For this review, take the finished solid that the model builds, in its own axes (mm). A direction names the side the tool comes from. Give positions to 0.01 mm unless a question says otherwise; leave off trailing zeros. Write each loop counter-clockwise with the first axis right and the second up, starting at its lowest first coordinate (ties: lowest second). Pieces come first, ordered by that corner, then holes. Notation, with made-up numbers: M 34,62.25 L 86,62.25 A13 ccw 86,87.25 Z; hole C 33.5,43 d4. An arc over 180 degrees is marked long. One line per item, written item: value. Start each with the question number.
Item 1: Clearance check with flat-ended pins moving along their axes: pin 1 Ø10 at (x, z) = (59, 13.5) entering from -Y; pin 2 Ø21 at (x, y) = (31, 34) entering from -Z. State where each tip first meets the part, or that it passes through.
Item 2: Consider section A-A, the plane z = -2. Write out the cut boundary in (x, y).
Item 3: Consider section B-B, the plane x = 44. Write out the cut boundary in (y, z).
Item 4: Mouldability with a two-part tool opening along X and no side actions: class faces 6 (the face through (7, 6, -0.5)), 7 (the face through (36, 38, 25)) as released by +X, released by -X, zero draft, split by the parting line, or undercut.
Item 5: Consider section D-D, the plane y = 11. Write out the cut boundary in (x, z), and give its area (3 significant figures).
Item 6: To check wall thickness, follow probe 1 along Y at (x, z) = (66, -0.25); probe 2 along Z at (x, y) = (60.5, 46.5); probe 3 along X at (y, z) = (58.5, 6.5). State the ranges of each line that lie inside material, in increasing order.
Item 7: Tool access review of faces 1 (the face through (37, 14.5, -4)), 2 (the face through (73, 5, 11)), 3 (the face through (37, 2, 11)), 4 (the face through (71.23, 7.74, -2.78)), 5 (the face through (11.707, 66.677, 24.014)): name each direction out of +Z, -Z, +X, -X, +Y, -Y from which nothing blocks a thin tool from reaching the whole face with its end or side.
```python
from build123d import *

# Parameters (mm, degrees)
SKETCH1_W           = 74
SKETCH1_H           = 74
BOSS_EXTRUDE1_DEPTH = 25
SHELL1_T            = -2
SKETCH2_W           = 8
SKETCH2_H           = 4.5
CUT_EXTRUDE1_DEPTH  = 22
SKETCH3_R           = 3.175
CUT_EXTRUDE2_DEPTH  = 108.596468344
SKETCH4_W           = 74
SKETCH4_H           = 74
BOSS_EXTRUDE2_DEPTH = 8
CUT_EXTRUDE3_START  = -3
CUT_EXTRUDE3_DEPTH  = 4.5
SKETCH6_W           = 45
SKETCH6_H           = 45
CUT_EXTRUDE4_DEPTH  = 8
CUT_EXTRUDE10_START = -1
CUT_EXTRUDE10_DEPTH = 1
SKETCH5_4_R         = 2
CUT_EXTRUDE11_DEPTH = 9


# Read off the part's stored shape, not the designer's step: Cut-Extrude10
with BuildPart() as part:
    # Sketch1 → Boss-Extrude1 (new body)
    with BuildSketch(Plane.XY):
        with Locations((37, 37)):
            Rectangle(SKETCH1_W, SKETCH1_H)
    extrude(amount=BOSS_EXTRUDE1_DEPTH)

    # Shell1
    shell1_openings = [part.faces().sort_by_distance(p)[0] for p in [
        (37, 37, 0),
    ]]
    offset(amount=SHELL1_T, openings=shell1_openings, kind=Kind.INTERSECTION)

    # Sketch2 → Cut-Extrude1 (cut)
    with BuildSketch(Plane(origin=(74, 0, 0), x_dir=(0, 0, -1), z_dir=(1, 0, 0))):
        with Locations((-11, 7.25)):
            Rectangle(SKETCH2_W, SKETCH2_H)
    extrude(amount=-CUT_EXTRUDE1_DEPTH, mode=Mode.SUBTRACT)

    # Sketch3 → Cut-Extrude2 (cut, through all)
    with BuildSketch(Plane.XY.offset(25)):
        with Locations((10, 64)):
            Circle(SKETCH3_R)
        with Locations((64, 10)):
            Circle(SKETCH3_R)
    extrude(amount=-CUT_EXTRUDE2_DEPTH, mode=Mode.SUBTRACT)

    # Sketch4 → Boss-Extrude2 (add)
    with BuildSketch(Plane(origin=(0, 0, 0), x_dir=(-1, 0, 0), z_dir=(0, 0, -1))):
        with Locations((-37, 37)):
            Rectangle(SKETCH4_W, SKETCH4_H)
    extrude(amount=BOSS_EXTRUDE2_DEPTH)

    # Sketch5 → Cut-Extrude3 (cut)
    with BuildSketch(Plane(origin=(0, 0, -8), x_dir=(-1, 0, 0), z_dir=(0, 0, -1)).offset(CUT_EXTRUDE3_START)):
        Polygon((-60.919317631, 8), (-63.459658816, 12.4), (-68.540341184, 12.4), (-74.568746864, 1.958495074), (-74.568746864, -0.972282173), (-66.099467159, -0.972282173), align=None)
        Polygon((-63.463624712, 61.59771267), (-60.919319694, 65.995421768), (-65.802792889, 74.471475085), (-74.465371111, 74.471475085), (-74.465371111, 71.879253606), (-68.544305018, 61.602290902), align=None)
        Polygon((-5.459702524, 61.599974765), (0.703595557, 72.274875291), (0.703595557, 74.471475085), (-8.189590882, 74.471475085), (-13.080682369, 66.00005047), (-10.540384893, 61.600025235), align=None)
        Polygon((-10.540490231, 12.399913945), (-13.080682366, 7.999827894), (-7.995582963, -0.807133653), (0.571776258, -0.807133653), (0.571776258, 1.953893119), (-5.459807865, 12.40008605), align=None)
    extrude(amount=-CUT_EXTRUDE3_DEPTH, mode=Mode.SUBTRACT)

    # Sketch6 → Cut-Extrude4 (cut)
    with BuildSketch(Plane(origin=(0, 0, -8), x_dir=(-1, 0, 0), z_dir=(0, 0, -1))):
        with Locations((-37, 37)):
            Rectangle(SKETCH6_W, SKETCH6_H)
    extrude(amount=-CUT_EXTRUDE4_DEPTH, mode=Mode.SUBTRACT)

    # Cut-Extrude10 outline → Cut-Extrude10 (cut)
    with BuildSketch(Plane.XZ.offset(CUT_EXTRUDE10_START)):
        with BuildLine():
            add(Edge.make_bspline(
                [(12.244921875, 14.608337696), (12.22296299, 14.60920838), (12.179368061, 14.610936947), (12.115469745, 14.625798621), (12.053855992, 14.648733433), (12.016469754, 14.671753524), (11.99765625, 14.683337696)],
                knots=[0, 0, 0, 0, 0.251074868, 0.498458438, 0.747614234, 1, 1, 1, 1], degree=3))
            add(Edge.make_bspline(
                [(12.45, 14.828650196), (12.44810186, 14.799147003), (12.444554554, 14.744010497), (12.402329284, 14.672042766), (12.332334145, 14.623910287), (12.275809653, 14.613840387), (12.244921875, 14.608337696)],
                knots=[0, 0, 0, 0, 0.262135661, 0.489887456, 0.721249278, 1, 1, 1, 1], degree=3))
            add(Edge.make_bspline(
                [(12.4078125, 14.970447071), (12.420108898, 14.947127329), (12.443588874, 14.902598273), (12.447931564, 14.852508226), (12.45, 14.828650196)],
                knots=[0, 0, 0, 0, 0.523697188, 1, 1, 1, 1], degree=3))
            Line((12.4078125, 14.970447071), (5.534765625, 21.851697071))
            Line((5.534765625, 21.851697071), (5.4609375, 21.882165821))
            add(Edge.make_bspline(
                [(5.1, 21.652478321), (5.101130742, 21.670561394), (5.103297124, 21.705206632), (5.119685049, 21.75396019), (5.149823147, 21.794252088), (5.190287736, 21.827525127), (5.242920358, 21.851708451), (5.305475941, 21.870670729), (5.379789996, 21.880316446), (5.432791747, 21.881524371), (5.4609375, 21.882165821)],
                knots=[0, 0, 0, 0, 0.112194147, 0.214952003, 0.313891338, 0.420689243, 0.536721732, 0.670960238, 0.825268571, 1, 1, 1, 1], degree=3))
            add(Edge.make_bspline(
                [(5.157421875, 21.525915821), (5.140627717, 21.547577619), (5.111281334, 21.585429794), (5.103379727, 21.632391539), (5.1, 21.652478321)],
                knots=[0, 0, 0, 0, 0.572273528, 1, 1, 1, 1], degree=3))
            Line((5.157421875, 21.525915821), (11.99765625, 14.683337696))
        make_face()
        with BuildLine():
            add(Edge.make_bspline(
                [(12.830859375, 16.332165821), (12.806611722, 16.332880637), (12.760653103, 16.334235487), (12.695606656, 16.343185504), (12.639038997, 16.359243561), (12.590419576, 16.382273546), (12.548696495, 16.410908541), (12.516703569, 16.448495353), (12.492316543, 16.491450489), (12.483699168, 16.523311237), (12.479296875, 16.539587696)],
                knots=[0, 0, 0, 0, 0.163241443, 0.30940526, 0.440897743, 0.557355848, 0.670469959, 0.778582052, 0.886885889, 1, 1, 1, 1], degree=3))
            Line((12.830859375, 16.332165821), (12.997265625, 16.332165821))
            add(Edge.make_bspline(
                [(13.065234375, 16.334509571), (13.054297092, 16.334112667), (13.031642253, 16.333290544), (13.008984624, 16.332549239), (12.997265625, 16.332165821)],
                knots=[0, 0, 0, 0, 0.482779122, 1, 1, 1, 1], degree=3))
            Line((13.065234375, 16.334509571), (13.15078125, 16.362634571))
            Line((13.15078125, 16.362634571), (13.454296875, 16.667322071))
            Line((13.454296875, 16.667322071), (13.491796875, 16.739978321))
            Line((13.491796875, 16.739978321), (13.5, 17.297790821))
            Line((13.5, 17.297790821), (13.5, 17.371618946))
            add(Edge.make_bspline(
                [(13.20234375, 17.944665821), (13.210597157, 17.929849426), (13.228545564, 17.897628712), (13.256314404, 17.845089826), (13.288074333, 17.78479063), (13.324465456, 17.717657372), (13.363157298, 17.642066218), (13.405143778, 17.558563248), (13.452185232, 17.468028061), (13.483699781, 17.404485145), (13.5, 17.371618946)],
                knots=[0, 0, 0, 0, 0.078785549, 0.171332276, 0.276048266, 0.395387691, 0.526054495, 0.670509549, 0.829578188, 1, 1, 1, 1], degree=3))
            Line((13.20234375, 17.944665821), (12.403125, 18.479040821))
            add(Edge.make_bspline(
                [(12.289453125, 18.507165821), (12.31084801, 18.5052121), (12.350224476, 18.501616352), (12.386540839, 18.486118184), (12.403125, 18.479040821)],
                knots=[0, 0, 0, 0, 0.543341929, 1, 1, 1, 1], degree=3))
            add(Edge.make_bspline(
                [(12.179296875, 18.494275196), (12.201126009, 18.497814185), (12.237664521, 18.503737892), (12.274588549, 18.506181923), (12.289453125, 18.507165821)],
                knots=[0, 0, 0, 0, 0.597428096, 1, 1, 1, 1], degree=3))
            add(Edge.make_bspline(
                [(12.005859375, 18.353650196), (12.012754805, 18.365403015), (12.028374155, 18.392025197), (12.067688375, 18.425310284), (12.117788217, 18.461646386), (12.157466096, 18.482694512), (12.179296875, 18.494275196)],
                knots=[0, 0, 0, 0, 0.179374527, 0.406314537, 0.673354122, 1, 1, 1, 1], degree=3))
            add(Edge.make_bspline(
                [(11.98828125, 18.276306446), (11.990007203, 18.287684739), (11.993981075, 18.31388238), (12.001567772, 18.339282172), (12.005859375, 18.353650196)],
                knots=[0, 0, 0, 0, 0.434325116, 1, 1, 1, 1], degree=3))
            add(Edge.make_bspline(
                [(12.084375, 18.115759571), (12.069768434, 18.129757216), (12.042992013, 18.155417378), (12.013246552, 18.197681646), (11.992279819, 18.236971695), (11.9895321, 18.264001579), (11.98828125, 18.276306446)],
                knots=[0, 0, 0, 0, 0.315523821, 0.578411003, 0.808079218, 1, 1, 1, 1], degree=3))
            Line((12.084375, 18.115759571), (12.778125, 17.652868946))
            Line((12.778125, 17.652868946), (12.975, 17.263806446))
            Line((12.975, 17.263806446), (12.975, 16.874743946))
            Line((12.975, 16.874743946), (12.891522636, 16.791266582))
            add(Edge.make_bspline(
                [(12.870703125, 16.792712696), (12.87764234, 16.792220225), (12.884581555, 16.791727755), (12.891522636, 16.791266582)],
                knots=[0, 0, 0, 0, 0.362748525, 0.362748525, 0.362748525, 0.362748525], degree=3))
            Line((12.870703125, 16.792712696), (12.805078125, 16.792712696))
            add(Edge.make_bspline(
                [(12.53671875, 16.698962696), (12.549147315, 16.713703314), (12.575814448, 16.745331261), (12.638752816, 16.772945663), (12.716162101, 16.790262491), (12.773683775, 16.791847581), (12.805078125, 16.792712696)],
                knots=[0, 0, 0, 0, 0.193970343, 0.416189066, 0.681365937, 1, 1, 1, 1], degree=3))
            add(Edge.make_bspline(
                [(12.479296875, 16.539587696), (12.481482036, 16.569008186), (12.48582524, 16.627484051), (12.51982501, 16.675235867), (12.53671875, 16.698962696)],
                knots=[0, 0, 0, 0, 0.503121942, 1, 1, 1, 1], degree=3))
        make_face()
    extrude(amount=CUT_EXTRUDE10_DEPTH, mode=Mode.SUBTRACT)

    # Sketch5<4> → Cut-Extrude11 (cut)
    with BuildSketch(Plane(origin=(0, 0, -8), x_dir=(-1, 0, 0), z_dir=(0, 0, -1))):
        with Locations((-66, 66)):
            Circle(SKETCH5_4_R)
        with Locations((-8, 66)):
            Circle(SKETCH5_4_R)
        with Locations((-8, 8)):
            Circle(SKETCH5_4_R)
        with Locations((-66, 8)):
            Circle(SKETCH5_4_R)
    extrude(amount=-CUT_EXTRUDE11_DEPTH, mode=Mode.SUBTRACT)


solid = part.part
```
Model answer:
1. pin 1: stops at y = 0
1. pin 2: stops at z = 23
2. outline: M 0,2.94 L 5.46,12.4 L 10.54,12.4 L 13.08,8 L 8.46,0 L 65.54,0 L 60.92,8 L 63.46,12.4 L 68.54,12.4 L 74,2.94 L 74,71.07 L 68.54,61.6 L 63.46,61.6 L 60.92,66 L 65.53,74 L 8.46,74 L 13.08,66 L 10.54,61.6 L 5.46,61.6 L 0,71.06 Z; hole M 14.5,14.5 L 59.5,14.5 L 59.5,59.5 L 14.5,59.5 Z
3. outline: M 0,-8 L 14.5,-8 L 14.5,0 L 2,0 L 2,23 L 72,23 L 72,0 L 59.5,0 L 59.5,-8 L 74,-8 L 74,25 L 0,25 Z
4. face 6: undercut
4. face 7: zero draft
5. outline: M 0,-8 L 74,-8 L 74,25 L 67.01,25 L 67.01,23 L 72,23 L 72,0 L 2,0 L 2,23 L 60.99,23 L 60.99,25 L 0,25 Z; hole M 4.65,-5 L 11.35,-5 L 11.35,-0.5 L 4.65,-0.5 Z; hole M 62.65,-5 L 69.35,-5 L 69.35,-0.5 L 62.65,-0.5 Z
5. area: 760 mm2
6. probe 1: y = 0 to 6, 10 to 64, 68 to 74
6. probe 2: z = -8 to 0, 23 to 25
6. probe 3: x = 0 to 2, 72 to 74
7. face 1: -Z
7. face 2: +X
7. face 3: none
7. face 4: -Y
7. face 5: +Z
